Autodesk Inventor part; units mm, degrees
ref_plane "YZ Plane" through (0, 0, 0) normal (1, 0, 0) x (0, 1, 0)
ref_plane "XZ Plane" through (0, 0, 0) normal (0, 1, 0) x (-1, 0, 0)
ref_plane "XY Plane" through (0, 0, 0) normal (0, 0, 1) x (1, 0, 0)
sketch "Sketch1" plane through (0, 0, 0) normal (0, 0, 1) x (1, 0, 0)
  arc A0 (5.5811, -56.8606) -> (20.209, -64.6836) centre (38.8796, -12.1848) ccw construction
  arc A1 (-7.6539, -43.4667) -> (5.5811, -56.8606) centre (37.8873, -11.7018) ccw construction
  arc A2 (-7.6539, -43.4667) -> (-31.2183, -12.0793) centre (-386.265, -303.1724) ccw construction
  arc A3 (-31.2183, -12.0793) -> (-63.3277, 19.0744) centre (-191.6112, -145.2692) ccw construction
  arc A4 (-67.5206, 26.3221) -> (-63.3277, 19.0744) centre (-54.6162, 28.9507) ccw construction
  arc A5 (-66.9469, 41.0059) -> (-67.5206, 26.3221) centre (-15.6776, 31.6496) ccw construction
  line L0 (-66.9469, 41.0059) -> (-50.7446, 56.9005) construction
  arc A6 (-3.6955, 79.7027) -> (-26.0985, 81.0785) centre (-17.6076, 36.2535) ccw construction
  arc A7 (1.4491, 74.6716) -> (-3.6955, 79.7027) centre (-6.1453, 72.0517) ccw construction
  arc A8 (2.6831, 69.1533) -> (1.4491, 74.6716) centre (-18.5892, 67.2935) ccw construction
  arc A9 (2.6831, 69.1533) -> (3.1898, 63.5624) centre (229.5421, 86.8959) ccw construction
  arc A10 (3.1898, 63.5624) -> (8.7161, 49.818) centre (30.4167, 66.5265) ccw construction
  arc A11 (8.7161, 49.818) -> (19.0471, 39.3259) centre (47.1297, 77.3097) ccw construction
  arc A12 (19.0471, 39.3259) -> (32.6891, 29.8296) centre (104.4845, 147.5139) ccw construction
  arc A13 (32.6891, 29.8296) -> (50.5655, 19.6706) centre (502.3948, 835.5524) ccw construction
  arc A14 (57.8671, 12.5741) -> (50.5655, 19.6706) centre (33.0101, -5.6965) ccw construction
  arc A15 (67.0572, -4.125) -> (57.8671, 12.5741) centre (18.4686, -19.9867) ccw construction
  arc A16 (68.9532, -23.0115) -> (67.0572, -4.125) centre (24.8632, -17.8992) ccw construction
  line L1 (-52.1723, 55.4999) -> (-51.76, 55.076) construction
  line L2 (43.4701, -39.9764) -> (43.0518, -39.5463) construction
  line L3 (42.0363, -41.3708) -> (43.4701, -39.9764) construction
  line L4 (-4.1456, -47.7345) -> (58.0182, 12.7211)
  line L5 (56.6239, 14.1548) -> (-5.54, -46.3007)
  line L6 (-55.3767, 12.3052) -> (3.7843, 69.8404)
  line L7 (2.3899, 71.2742) -> (-56.7711, 13.739)
  line L8 (-56.7711, 13.739) -> (-55.3767, 12.3052)
  line L9 (2.3899, 71.2742) -> (3.7843, 69.8404)
  line L10 (-52.1723, 55.4999) -> (-50.7446, 56.9005) construction
  line L11 (-4.1456, -47.7345) -> (-5.54, -46.3007)
  line L12 (58.0182, 12.7211) -> (56.6239, 14.1548)
  line L13 (-51.76, 55.076) -> (-50.3262, 56.4704)
  line L14 (41.618, -40.9406) -> (43.0518, -39.5463)
  line L15 (-51.76, 55.076) -> (41.618, -40.9406)
  line L16 (-50.3262, 56.4704) -> (-50.7446, 56.9005) construction
  line L17 (-50.7446, 56.9005) -> (-26.0985, 81.0785) construction
  line L18 (43.0518, -39.5463) -> (-50.3262, 56.4704)
  line L19 (41.618, -40.9406) -> (42.0363, -41.3708) construction
  point P0 (0, 0)
  point P1 (-8.2693, 4.2237)
  point P2 (-4.9861, 4.7501)
  point P3 (-66.0155, 22.3561)
  point P4 (24.203, -20.1649)
  point P5 (22.8086, -18.7311)
  point P6 (-30.7071, 36.2969)
  point P7 (-32.1015, 37.7306)
  point P8 (-33.5353, 36.3363)
  point P9 (-32.1409, 34.9025)
  point P10 (21.3749, -20.1255)
  point P11 (22.7692, -21.5593)
  point P12 (22.8086, -18.7311)
  point P13 (-30.7071, 36.2969)
  point P14 (-32.1409, 34.9025)
  point P15 (21.3749, -20.1255)
  point P16 (24.203, -20.1649)
  point P17 (22.7692, -21.5593)
  point P18 (-33.5353, 36.3363)
  point P19 (-32.1015, 37.7306)
  dimension "d244" = 2
  dimension "d245" = 2
  dimension "d251" = 0.6
  dimension "d252" = 0.6
  dimension "d253" = 2
extrude "Extrusion12" add sketch "Sketch1" along normal blind 2
move faces "Move1" translate (1.7922, 1.743, 0) faces at (3.3195, 70.3184, 0.6667)
move faces "Move2" translate (1.7922, 1.743, 0) faces at (57.5534, 13.199, 0.6667)
move faces "Move3" translate (-1.7922, -1.743, 0) faces at (-4.6104, -47.2565, 1.3333)
move faces "Move4" translate (-1.7922, -1.743, 0) faces at (-56.3063, 13.2611, 0.6667)
move faces "Move5" translate (-2.1613, 2.2224, 0) faces at (-50.8042, 56.0056, 0.6667)
move faces "Move6" translate (2.4402, -2.5091, 0) faces at (42.0959, -40.4758, 0.6667)
properties part number "print009_Guss_innen_erweitert"
Check sheet for the modelled part. Datum: model origin and axes. Units: mm. A direction names the side the tool comes from. Give positions to 0.01 mm unless a question says otherwise; leave off trailing zeros. Loops run counter-clockwise (first coordinate to the right, second up) from the corner with the lowest first, then second, coordinate; pieces in that order, holes last. Notation, with made-up numbers: M 78,-17 L 132,-17 A18 ccw 132,18 Z; hole C 19.25,-21.5 d9. An arc over 180 degrees is marked long. Use a Markdown table: item, result. Add a question column.
Q1. Sectioned sample at C-C, the plane y = 30.5. Record the cut outline in (x, z).
Q2. Tool access check on faces 4 (the flat face through (7.22, -33.89, 0.99)), 5 (the flat face through (41.76, -3.09, 0.99)), 6 (the flat face through (33.265, -32.351, 0.986)), 7 (the flat face through (-3.575, 8.398, 0.986)). Record the directions out of +Z, -Z, +X, -X, +Y, -Y that give a thin tool (end or side, any length) a straight path to the whole face; none if there is none.
Q3. Mould release check, pull along Y, two halves, no side actions. Record for faces 1 (the flat face through (-43.871, 46.964, 0.986)), 2 (the flat face through (-4, 8, 2)), 3 (the flat face through (40.862, -1.174, 0.986)): pulls with the +Y half, pulls with the -Y half, needs draft (parallel to the pull), parting line crosses it, or undercut.
Q4. Sectioned sample at B-B, the plane z = 1.65. Record the cut outline in (x, y).
Q5. Scan lines: line 1 along Y through (x, z) = (-5, 0.4); line 2 along X through (y, z) = (14, 0.6); line 3 along X through (y, z) = (-30, 1.6). Record each from-to range of solid material in increasing order. Write a range as [from, to].
Q6. Sectioned sample at A-A, the plane x = -21. Record the cut outline in (y, z), then the cut area to 3 significant figures.
Verdict:
| question | item | result |
|---|---|---|
| 1 | outline | M -39.54,0 L -36.67,0 L -36.67,2 L -39.54,2 Z; M -27.86,0 L -25.07,0 L -25.07,2 L -27.86,2 Z |
| 2 | face 4 | +Z, -Z, -X |
| 2 | face 5 | +Z, -Z, +X |
| 2 | face 6 | +Z, -Z, -Y |
| 2 | face 7 | +Z, -Z |
| 3 | face 1 | undercut |
| 3 | face 2 | needs draft |
| 3 | face 3 | pulls with the +Y half |
| 4 | outline | M -58.56,12 L -57.17,10.56 L -32.14,34.9 L 21.37,-20.13 L -7.33,-48.04 L -5.94,-49.48 L 22.77,-21.56 L 44.06,-43.45 L 45.49,-42.06 L 24.2,-20.16 L 59.81,14.46 L 58.42,15.9 L 22.81,-18.73 L -30.71,36.3 L 5.58,71.58 L 4.18,73.02 L -32.1,37.73 L -52.49,58.69 L -53.92,57.3 L -33.54,36.34 Z |
| 5 | line 1 | [-48.57, -45.78], [6.99, 9.86], [61.3, 64.09] |
| 5 | line 2 | [-56.5, -53.63], [-11.81, -9.02], [56.46, 59.33] |
| 5 | line 3 | [11.22, 14.09], [30.98, 33.77] |
| 6 | outline | M 23.45,0 L 26.32,0 L 26.32,2 L 23.45,2 Z; M 45.74,0 L 48.53,0 L 48.53,2 L 45.74,2 Z |
| 6 | area | 11.3 mm^2 |
